Autodesk Fusion 360 part; units mm, degrees
sketch "Sketch1" plane through (0, 0, 0) normal (0, 1, 0) x (1, 0, 0)
  circle A0 centre (0, 0) radius 10.5
  dimension "d1" = 21
extrude "Extrude1" add sketch "Sketch1" along normal blind 17
sketch "Sketch2" plane through (0, 0, 0) normal (0, -1, 0) x (1, 0, 0)
  circle A0 centre (0, 0) radius 10.5
  circle A1 centre (0, 0) radius 13
  dimension "d4" = 26
extrude "Extrude2" add sketch "Sketch2" along normal blind 3 contours A0 | A1
sketch "Sketch3" plane through (0, 17, 0) normal (0, 1, 0) x (-1, 0, 0)
  circle A0 centre (0, 0) radius 10.5
  circle A1 centre (0, 0) radius 13
  dimension "d7" = 26
extrude "Extrude3" add sketch "Sketch3" along normal blind 3 contours A0 | A1
sketch "Sketch4" plane through (0, -3, 0) normal (0, -1, 0) x (1, 0, 0)
  circle A0 centre (0, 0) radius 13
  circle A1 centre (0, 0) radius 1.05
  dimension "d10" = 2.1
extrude "Extrude4" cut sketch "Sketch4" against normal blind 6 contours A1
Check sheet for the modelled part. Datum: model origin and axes. Units: mm. A direction names the side the tool comes from. Round coordinates to 2 decimals unless told otherwise and drop trailing zeros. Loops run counter-clockwise (first coordinate to the right, second up) from the corner with the lowest first, then second, coordinate; pieces in that order, holes last.
1. Scan lines: probe 1 along Y at (x, z) = (1.75, -10.5); probe 2 along Z at (x, y) = (0, -1.35); probe 3 along Z at (x, y) = (0, 0.2). Record each from-to range of solid material in increasing order.
2. Set-up check for faces 5 (the flat face through (9, 17, 6)), 6 (the cylindrical face through (-10.316, -1.479, 7.91)): record each of +Z, -Z, +X, -X, +Y, -Y from which the full face is reachable in a straight line by a thin tool's end or side.
3. Sectioned sample at A-A on z = 0. Record the boundary of the cut face in (x, y).
4. Sectioned sample at B-B on x = 0. Record the boundary of the cut face in (y, z), and give its area (3 significant figures).
5. Gauge pin test, flat ends, axial feed: pin 1 Ø6 at (x, y) = (-2, 11) entering from -Z; pin 2 Ø1 at (y, z) = (2.5, -8) entering from -X; pin 3 Ø8 at (y, z) = (9, -3.5) entering from +X. Record the tip position at first contact, or that the pin passes through.
6. Mould release check, pull along Z, two halves, no side actions. Record for faces 1 (the flat face through (0, 3, 0)), 2 (the flat face through (3, -3, 0)), 3 (the cylindrical face through (1, -0.04, 0.32)), 4 (the cylindrical face through (10, 8.4, 3.2)): released by +Z, released by -Z, zero draft, split by the parting line, or undercut.
7. Sectioned sample at C-C on y = 5. Record the boundary of the cut face in (x, z), and give its area (3 significant figures).
8. Sectioned sample at D-D on z = 3. Record the boundary of the cut face in (x, y), and give its area (3 significant figures).
Recorded:
1. probe 1: y = -3 to 0, 17 to 20
1. probe 2: z = -13 to -1.05, 1.05 to 13
1. probe 3: z = -10.5 to -1.05, 1.05 to 10.5
2. face 5: none
2. face 6: +Y, -Y
3. outline: (-13, -3) - (-1.05, -3) - (-1.05, 3) - (1.05, 3) - (1.05, -3) - (13, -3) - (13, 0) - (10.5, 0) - (10.5, 17) - (13, 17) - (13, 20) - (-13, 20) - (-13, 17) - (-10.5, 17) - (-10.5, 0) - (-13, 0) - close
4. outline: (-3, -13) - (0, -13) - (0, -10.5) - (17, -10.5) - (17, -13) - (20, -13) - (20, 13) - (17, 13) - (17, 10.5) - (0, 10.5) - (0, 13) - (-3, 13) - (-3, 1.05) - (3, 1.05) - (3, -1.05) - (-3, -1.05) - close
4. area: 500 mm2
5. pin 1: stops at z = -10.5
5. pin 2: stops at x = -7.35
5. pin 3: stops at x = 10.5
6. face 1: undercut
6. face 2: zero draft
6. face 3: undercut
6. face 4: split by the parting line
7. outline: circle Ø21 at (0, 0)
7. area: 346 mm2
8. outline: (-12.65, -3) - (12.65, -3) - (12.65, 0) - (10.06, 0) - (10.06, 17) - (12.65, 17) - (12.65, 20) - (-12.65, 20) - (-12.65, 17) - (-10.06, 17) - (-10.06, 0) - (-12.65, 0) - close
8. area: 494 mm2
